from build123d import *

# Parameters (mm, degrees)
SKETCH1_W           = 228.6
SKETCH1_H           = 101.6
BOSS_EXTRUDE1_DEPTH = 6.35
CUT_EXTRUDE1_DEPTH  = 76.2
SKETCH3_W           = 6.35
SKETCH3_H           = 25.4
BOSS_EXTRUDE2_DEPTH = 76.2
SKETCH5_W           = 6.35
SKETCH5_H           = 6.35
BOSS_EXTRUDE3_DEPTH = 63.5
SKETCH6_W           = 6.35
SKETCH6_H           = 6.35
BOSS_EXTRUDE4_DEPTH = 63.5
SKETCH7_R           = 0.79375
CUT_EXTRUDE3_DEPTH  = 50.8


with BuildPart() as part:
    # Sketch1 → Boss-Extrude1 (new body)
    with BuildSketch(Plane.XY):
        with Locations((114.3, 50.8)):
            Rectangle(SKETCH1_W, SKETCH1_H)
    extrude(amount=BOSS_EXTRUDE1_DEPTH)

    # Sketch2 → Cut-Extrude1 (cut)
    with BuildSketch(Plane.XY.offset(6.35)):
        with BuildLine():
            ThreePointArc((119.0625, 50.8), (158.75, 11.1125), (198.4375, 50.8))
            Line((198.4375, 50.8), (119.0625, 50.8))
        make_face()
        with BuildLine():
            Line((119.0625, 50.8), (198.4375, 50.8))
            ThreePointArc((198.4375, 50.8), (158.75, 90.4875), (119.0625, 50.8))
        make_face()
    extrude(amount=-CUT_EXTRUDE1_DEPTH, mode=Mode.SUBTRACT)

    # Sketch3 → Boss-Extrude2 (add)
    with BuildSketch(Plane(origin=(228.6, 0, 0), x_dir=(0, 0, -1), z_dir=(1, 0, 0))):
        with Locations((-3.175, 50.8)):
            Rectangle(SKETCH3_W, SKETCH3_H)
    extrude(amount=BOSS_EXTRUDE2_DEPTH)

    # Sketch5 → Boss-Extrude3 (add)
    with BuildSketch(Plane(origin=(0, 63.5, 0), x_dir=(1, 0, 0), z_dir=(0, 1, 0))):
        with Locations((231.775, -3.175)):
            Rectangle(SKETCH5_W, SKETCH5_H)
    extrude(amount=BOSS_EXTRUDE3_DEPTH)

    # Sketch6 → Boss-Extrude4 (add)
    with BuildSketch(Plane.XZ.offset(-38.1)):
        with Locations((231.775, 3.175)):
            Rectangle(SKETCH6_W, SKETCH6_H)
    extrude(amount=BOSS_EXTRUDE4_DEPTH)

    # Sketch7 → Cut-Extrude3 (cut)
    with BuildSketch(Plane.XY.offset(6.35)):
        with Locations(Location((59.53125, 50.8, 0), (0, 0, 180))):
            Circle(SKETCH7_R)
        with Locations((59.53125, 79.375)):
            Circle(SKETCH7_R)
        with Locations(Location((88.10625, 50.8, 0), (0, 0, 180))):
            Circle(SKETCH7_R)
        with Locations((59.53125, 38.1)):
            Circle(SKETCH7_R)
        with Locations((30.95625, 50.8)):
            Circle(SKETCH7_R)
        with Locations((50.00625, 50.8)):
            Circle(SKETCH7_R)
        with Locations(Location((59.53125, 63.5, 0), (0, 0, 180))):
            Circle(SKETCH7_R)
        with Locations(Location((78.58125, 50.8, 0), (0, 0, 180))):
            Circle(SKETCH7_R)
        with Locations(Location((59.53125, 22.225, 0), (0, 0, 180))):
            Circle(SKETCH7_R)
        with Locations(Location((97.63125, 50.8, 0), (0, 0, 180))):
            Circle(SKETCH7_R)
        with Locations((21.43125, 50.8)):
            Circle(SKETCH7_R)
        with Locations((69.05625, 79.375)):
            Circle(SKETCH7_R)
        with Locations((40.48125, 50.8)):
            Circle(SKETCH7_R)
        with Locations(Location((69.05625, 63.5, 0), (0, 0, 180))):
            Circle(SKETCH7_R)
        with Locations(Location((69.05625, 50.8, 0), (0, 0, 180))):
            Circle(SKETCH7_R)
        with Locations((69.05625, 38.1)):
            Circle(SKETCH7_R)
        with Locations(Location((69.05625, 22.225, 0), (0, 0, 180))):
            Circle(SKETCH7_R)
        with Locations((78.58125, 79.375)):
            Circle(SKETCH7_R)
        with Locations(Location((78.58125, 63.5, 0), (0, 0, 180))):
            Circle(SKETCH7_R)
        with Locations((78.58125, 38.1)):
            Circle(SKETCH7_R)
        with Locations(Location((78.58125, 22.225, 0), (0, 0, 180))):
            Circle(SKETCH7_R)
        with Locations((88.10625, 79.375)):
            Circle(SKETCH7_R)
        with Locations(Location((88.10625, 63.5, 0), (0, 0, 180))):
            Circle(SKETCH7_R)
        with Locations((88.10625, 38.1)):
            Circle(SKETCH7_R)
        with Locations(Location((88.10625, 22.225, 0), (0, 0, 180))):
            Circle(SKETCH7_R)
        with Locations((97.63125, 79.375)):
            Circle(SKETCH7_R)
        with Locations(Location((97.63125, 63.5, 0), (0, 0, 180))):
            Circle(SKETCH7_R)
        with Locations((97.63125, 38.1)):
            Circle(SKETCH7_R)
        with Locations(Location((97.63125, 22.225, 0), (0, 0, 180))):
            Circle(SKETCH7_R)
        with Locations((21.43125, 22.225)):
            Circle(SKETCH7_R)
        with Locations(Location((21.43125, 38.1, 0), (0, 0, 180))):
            Circle(SKETCH7_R)
        with Locations((21.43125, 63.5)):
            Circle(SKETCH7_R)
        with Locations(Location((21.43125, 79.375, 0), (0, 0, 180))):
            Circle(SKETCH7_R)
        with Locations((30.95625, 22.225)):
            Circle(SKETCH7_R)
        with Locations(Location((30.95625, 38.1, 0), (0, 0, 180))):
            Circle(SKETCH7_R)
        with Locations((30.95625, 63.5)):
            Circle(SKETCH7_R)
        with Locations(Location((30.95625, 79.375, 0), (0, 0, 180))):
            Circle(SKETCH7_R)
        with Locations((40.48125, 22.225)):
            Circle(SKETCH7_R)
        with Locations(Location((40.48125, 38.1, 0), (0, 0, 180))):
            Circle(SKETCH7_R)
        with Locations((40.48125, 63.5)):
            Circle(SKETCH7_R)
        with Locations(Location((40.48125, 79.375, 0), (0, 0, 180))):
            Circle(SKETCH7_R)
        with Locations((50.00625, 22.225)):
            Circle(SKETCH7_R)
        with Locations(Location((50.00625, 38.1, 0), (0, 0, 180))):
            Circle(SKETCH7_R)
        with Locations((50.00625, 63.5)):
            Circle(SKETCH7_R)
        with Locations(Location((50.00625, 79.375, 0), (0, 0, 180))):
            Circle(SKETCH7_R)
    extrude(amount=-CUT_EXTRUDE3_DEPTH, mode=Mode.SUBTRACT)


solid = part.part
Geometry: final body of the model. Coordinates: model frame, mm. A direction names the side the tool comes from. Coordinates: 2 decimals unless noted, no trailing zeros. Loops run counter-clockwise (first coordinate to the right, second up) from the corner with the lowest first, then second, coordinate; pieces in that order, holes last. Notation, with made-up numbers: (62, 11) - (103, 11) arc R23 ccw to (103, 35) - close; hole circle Ø6 at (83.5, -32). An arc over 180 degrees is marked (long way). One line per question, with ' | ' between items. Start each with the question number.
(1) Cut plane A-A on x = 158.75. Output: boundary loops of the cut face in (y, z), and give its area (3 significant figures).
(2) Cut plane B-B on y = 70. Output: boundary loops of the cut face in (x, z), and give its area (3 significant figures).
(3) Ray query, L1, parallel to Y at x = 96.5, z = 2.75; L2, parallel to Y at x = 286, z = 1.5; L3, parallel to X at y = 94, z = 4. Return the intervals inside material, ascending. Write a range as from..to.
(4) Reachability of faces 1 (the flat face through (234.95, 95, 3)), 2 (the flat face through (113, 101.6, 3)), 3 (the flat face through (228.6, -13, 3)) from +Z, -Z, +X, -X, +Y, -Y: full face, straight path, thin tool, end or side. Return the list, or none.
(5) Cut plane D-D on x = 108.5. Output: boundary loops of the cut face in (y, z).
(6) Draft query along X for faces 4 (the flat face through (304.8, 51, 3)), 5 (the flat face through (232, 127, 3)), 6 (the cylindrical face through (196.605, 62.721, 3.219)). Return one class per face: +X half, -X half, draft (parallel to the pull), parting line (faces both ways), or undercut.
(7) First-contact query: pin 1 (1 mm diameter, centred on x = 97.63, y = 63.5, fed in from +Z); pin 2 (3 mm diameter, centred on x = 150, z = 2, fed in from -Y). Flat tips, straight axial feed; report the tip coordinate or a pass-through.
(8) Cut plane C-C on z = 2.25. Count the separate pieces of the cut face and the enclosed holes in it, and give its area (3 significant figures).
Here are the results:
1) outline: (0, 0) - (11.11, 0) - (11.11, 6.35) - (0, 6.35) - close; (90.49, 0) - (101.6, 0) - (101.6, 6.35) - (90.49, 6.35) - close | area: 141 mm²
2) outline: (0, 0) - (124.02, 0) - (124.02, 6.35) - (0, 6.35) - close; (193.48, 0) - (234.95, 0) - (234.95, 6.35) - (193.48, 6.35) - close | area: 1,050 mm²
3) L1: 0..101.6 | L2: 38.1..63.5 | L3: 0..234.95
4) face 1: +Z, -Z, +X, +Y | face 2: +Z, -Z, -X, +Y | face 3: +Z, -Z, -X, -Y
5) outline: (0, 0) - (101.6, 0) - (101.6, 6.35) - (0, 6.35) - close
6) face 4: +X half | face 5: draft | face 6: undercut
7) pin 1: through | pin 2: y = 0
8) separate pieces: 1 | enclosed holes: 46 | area: 20,900 mm²
